Verification items for the finished model (mm, model axes). Coordinates: 2 decimals unless noted, no trailing zeros. Order: outer loops, then holes, each group sorted by start corner. A loop starts at its lowest first (then second) coordinate and runs counter-clockwise, first axis right, second up.
Q1. Cross-section at A-A, the plane x = 366. Record the boundary of the cut face in (y, z), and give its area (3 significant figures).
Q2. Depth check by flat-ended pin: P1, Ø10, axis at x = 374, y = 56.5, coming from the +Z side. Enter the tip coordinate at first touch or a pass-through.
Q3. Thickness scan on line 1 (Y direction, x = 411.5, z = 19.55). Record the ranges inside material, lowest first.
Q4. Cross-section at B-B, the plane y = 110.5. Count the separate pieces of the cut face and the enclosed holes in it, and give its area (3 significant figures).
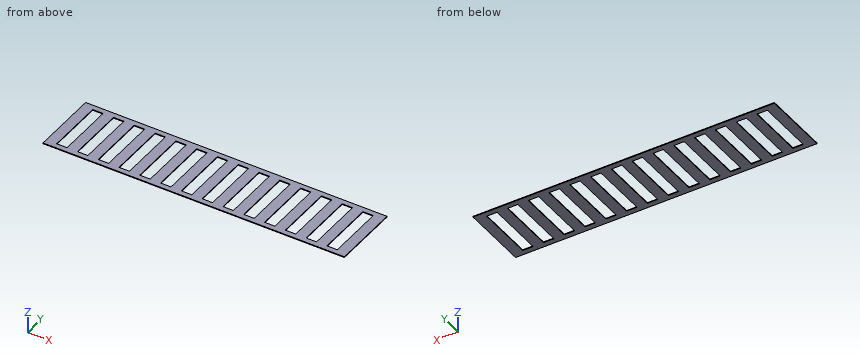
from build123d import *

# Parameters (mm, degrees)
TOPPING_PLINT_IZGARA_PANELI_1_START  = 18.5
SKETCH1_W                            = 580
SKETCH1_H                            = 130
TOPPING_PLINT_IZGARA_PANELI_1_DEPTH  = 1.5
TOPPING_PLINT_IZGARA_PANELI_2_START  = 17
SKETCH2_W                            = 20
SKETCH2_H                            = 110
TOPPING_PLINT_IZGARA_PANELI_2_DEPTH  = 4
TOPPING_PLINT_IZGARA_PANELI_3_START  = 17
SKETCH3_W                            = 20
SKETCH3_H                            = 110
TOPPING_PLINT_IZGARA_PANELI_3_DEPTH  = 4
TOPPING_PLINT_IZGARA_PANELI_4_START  = 17
SKETCH4_W                            = 20
SKETCH4_H                            = 110
TOPPING_PLINT_IZGARA_PANELI_4_DEPTH  = 4
TOPPING_PLINT_IZGARA_PANELI_5_START  = 17
SKETCH5_W                            = 20
SKETCH5_H                            = 110
TOPPING_PLINT_IZGARA_PANELI_5_DEPTH  = 4
TOPPING_PLINT_IZGARA_PANELI_6_START  = 17
SKETCH6_W                            = 20
SKETCH6_H                            = 110
TOPPING_PLINT_IZGARA_PANELI_6_DEPTH  = 4
TOPPING_PLINT_IZGARA_PANELI_7_START  = 17
SKETCH7_W                            = 20
SKETCH7_H                            = 110
TOPPING_PLINT_IZGARA_PANELI_7_DEPTH  = 4
TOPPING_PLINT_IZGARA_PANELI_8_START  = 17
SKETCH8_W                            = 20
SKETCH8_H                            = 110
TOPPING_PLINT_IZGARA_PANELI_8_DEPTH  = 4
TOPPING_PLINT_IZGARA_PANELI_9_START  = 17
SKETCH9_W                            = 20
SKETCH9_H                            = 110
TOPPING_PLINT_IZGARA_PANELI_9_DEPTH  = 4
TOPPING_PLINT_IZGARA_PANELI_10_START = 17
SKETCH10_W                           = 20
SKETCH10_H                           = 110
TOPPING_PLINT_IZGARA_PANELI_10_DEPTH = 4
TOPPING_PLINT_IZGARA_PANELI_11_START = 17
SKETCH11_W                           = 20
SKETCH11_H                           = 110
TOPPING_PLINT_IZGARA_PANELI_11_DEPTH = 4
TOPPING_PLINT_IZGARA_PANELI_12_START = 17
SKETCH12_W                           = 20
SKETCH12_H                           = 110
TOPPING_PLINT_IZGARA_PANELI_12_DEPTH = 4
TOPPING_PLINT_IZGARA_PANELI_13_START = 17
SKETCH13_W                           = 20
SKETCH13_H                           = 110
TOPPING_PLINT_IZGARA_PANELI_13_DEPTH = 4
TOPPING_PLINT_IZGARA_PANELI_14_START = 17
SKETCH14_W                           = 20
SKETCH14_H                           = 110
TOPPING_PLINT_IZGARA_PANELI_14_DEPTH = 4
TOPPING_PLINT_IZGARA_PANELI_15_START = 17
SKETCH15_W                           = 20
SKETCH15_H                           = 110
TOPPING_PLINT_IZGARA_PANELI_15_DEPTH = 4


with BuildPart() as part:
    # Sketch1 → TOPPING_plint_izgara_paneli_1 (new body)
    with BuildSketch(Plane.XY.offset(TOPPING_PLINT_IZGARA_PANELI_1_START)):
        with Locations((350, 105)):
            Rectangle(SKETCH1_W, SKETCH1_H)
    extrude(amount=TOPPING_PLINT_IZGARA_PANELI_1_DEPTH)

    # Sketch2 → TOPPING_plint_izgara_paneli_2 (cut)
    with BuildSketch(Plane.XY.offset(TOPPING_PLINT_IZGARA_PANELI_2_START)):
        with Locations((90, 105)):
            Rectangle(SKETCH2_W, SKETCH2_H)
    extrude(amount=TOPPING_PLINT_IZGARA_PANELI_2_DEPTH, mode=Mode.SUBTRACT)

    # Sketch3 → TOPPING_plint_izgara_paneli_3 (cut)
    with BuildSketch(Plane.XY.offset(TOPPING_PLINT_IZGARA_PANELI_3_START)):
        with Locations((130, 105)):
            Rectangle(SKETCH3_W, SKETCH3_H)
    extrude(amount=TOPPING_PLINT_IZGARA_PANELI_3_DEPTH, mode=Mode.SUBTRACT)

    # Sketch4 → TOPPING_plint_izgara_paneli_4 (cut)
    with BuildSketch(Plane.XY.offset(TOPPING_PLINT_IZGARA_PANELI_4_START)):
        with Locations((170, 105)):
            Rectangle(SKETCH4_W, SKETCH4_H)
    extrude(amount=TOPPING_PLINT_IZGARA_PANELI_4_DEPTH, mode=Mode.SUBTRACT)

    # Sketch5 → TOPPING_plint_izgara_paneli_5 (cut)
    with BuildSketch(Plane.XY.offset(TOPPING_PLINT_IZGARA_PANELI_5_START)):
        with Locations((210, 105)):
            Rectangle(SKETCH5_W, SKETCH5_H)
    extrude(amount=TOPPING_PLINT_IZGARA_PANELI_5_DEPTH, mode=Mode.SUBTRACT)

    # Sketch6 → TOPPING_plint_izgara_paneli_6 (cut)
    with BuildSketch(Plane.XY.offset(TOPPING_PLINT_IZGARA_PANELI_6_START)):
        with Locations((250, 105)):
            Rectangle(SKETCH6_W, SKETCH6_H)
    extrude(amount=TOPPING_PLINT_IZGARA_PANELI_6_DEPTH, mode=Mode.SUBTRACT)

    # Sketch7 → TOPPING_plint_izgara_paneli_7 (cut)
    with BuildSketch(Plane.XY.offset(TOPPING_PLINT_IZGARA_PANELI_7_START)):
        with Locations((290, 105)):
            Rectangle(SKETCH7_W, SKETCH7_H)
    extrude(amount=TOPPING_PLINT_IZGARA_PANELI_7_DEPTH, mode=Mode.SUBTRACT)

    # Sketch8 → TOPPING_plint_izgara_paneli_8 (cut)
    with BuildSketch(Plane.XY.offset(TOPPING_PLINT_IZGARA_PANELI_8_START)):
        with Locations((330, 105)):
            Rectangle(SKETCH8_W, SKETCH8_H)
    extrude(amount=TOPPING_PLINT_IZGARA_PANELI_8_DEPTH, mode=Mode.SUBTRACT)

    # Sketch9 → TOPPING_plint_izgara_paneli_9 (cut)
    with BuildSketch(Plane.XY.offset(TOPPING_PLINT_IZGARA_PANELI_9_START)):
        with Locations((370, 105)):
            Rectangle(SKETCH9_W, SKETCH9_H)
    extrude(amount=TOPPING_PLINT_IZGARA_PANELI_9_DEPTH, mode=Mode.SUBTRACT)

    # Sketch10 → TOPPING_plint_izgara_paneli_10 (cut)
    with BuildSketch(Plane.XY.offset(TOPPING_PLINT_IZGARA_PANELI_10_START)):
        with Locations((410, 105)):
            Rectangle(SKETCH10_W, SKETCH10_H)
    extrude(amount=TOPPING_PLINT_IZGARA_PANELI_10_DEPTH, mode=Mode.SUBTRACT)

    # Sketch11 → TOPPING_plint_izgara_paneli_11 (cut)
    with BuildSketch(Plane.XY.offset(TOPPING_PLINT_IZGARA_PANELI_11_START)):
        with Locations((450, 105)):
            Rectangle(SKETCH11_W, SKETCH11_H)
    extrude(amount=TOPPING_PLINT_IZGARA_PANELI_11_DEPTH, mode=Mode.SUBTRACT)

    # Sketch12 → TOPPING_plint_izgara_paneli_12 (cut)
    with BuildSketch(Plane.XY.offset(TOPPING_PLINT_IZGARA_PANELI_12_START)):
        with Locations((490, 105)):
            Rectangle(SKETCH12_W, SKETCH12_H)
    extrude(amount=TOPPING_PLINT_IZGARA_PANELI_12_DEPTH, mode=Mode.SUBTRACT)

    # Sketch13 → TOPPING_plint_izgara_paneli_13 (cut)
    with BuildSketch(Plane.XY.offset(TOPPING_PLINT_IZGARA_PANELI_13_START)):
        with Locations((530, 105)):
            Rectangle(SKETCH13_W, SKETCH13_H)
    extrude(amount=TOPPING_PLINT_IZGARA_PANELI_13_DEPTH, mode=Mode.SUBTRACT)

    # Sketch14 → TOPPING_plint_izgara_paneli_14 (cut)
    with BuildSketch(Plane.XY.offset(TOPPING_PLINT_IZGARA_PANELI_14_START)):
        with Locations((570, 105)):
            Rectangle(SKETCH14_W, SKETCH14_H)
    extrude(amount=TOPPING_PLINT_IZGARA_PANELI_14_DEPTH, mode=Mode.SUBTRACT)

    # Sketch15 → TOPPING_plint_izgara_paneli_15 (cut)
    with BuildSketch(Plane.XY.offset(TOPPING_PLINT_IZGARA_PANELI_15_START)):
        with Locations((610, 105)):
            Rectangle(SKETCH15_W, SKETCH15_H)
    extrude(amount=TOPPING_PLINT_IZGARA_PANELI_15_DEPTH, mode=Mode.SUBTRACT)


solid = part.part
Check values:
1. outline: (40, 18.5) - (50, 18.5) - (50, 20) - (40, 20) - close; (160, 18.5) - (170, 18.5) - (170, 20) - (160, 20) - close
1. area: 30.0 mm2
2. P1: passes through
3. line 1: y = 40 to 50, 160 to 170
4. separate pieces: 15
4. enclosed holes: 0
4. area: 450 mm2
